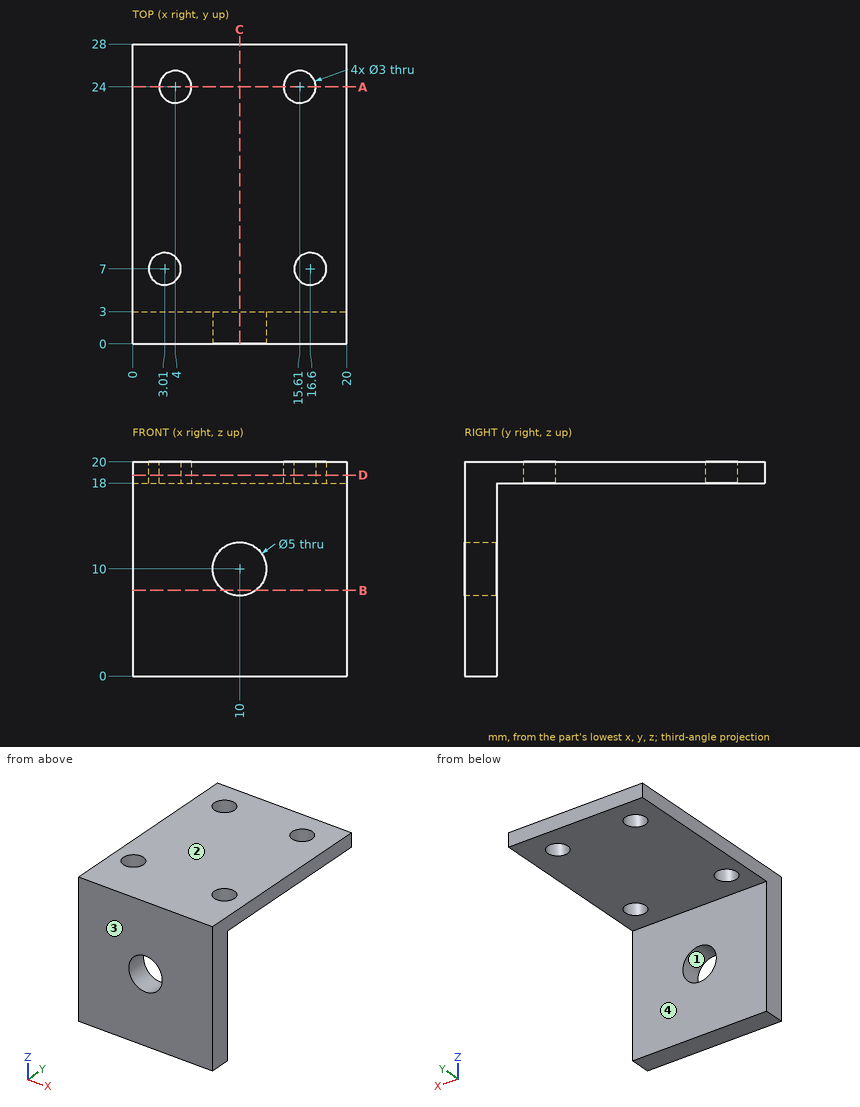
Design review of the part shown in the three views and the two pictorial views. Dimensions are in mm from the part's minimum x, y and z. A direction names the side the tool comes from. Coordinates: 2 decimals unless noted, no trailing zeros. Write each loop counter-clockwise with the first axis right and the second up, starting at its lowest first coordinate (ties: lowest second). Pieces come first, ordered by that corner, then holes. Notation, with made-up numbers: (-17, 59) -> (-7, 59) arc R16 cw to (-7, 81) -> close; hole circle Ø5 at (25.25, 76). An arc over 180 degrees is marked (long way). Answer in a Markdown table with one row per item.
1. Wall thickness on probe 1 along Y at (x, z) = (16.6, 18.65); probe 2 along X at (y, z) = (2.2, 10); probe 3 along Z at (x, y) = (3.5, 15): over which ranges is each line inside the solid? List them lowest first. Write a range as [from, to].
Answers below:
| item | result |
|---|---|
| probe 1 | y = [0, 5.5], [8.5, 22.87], [25.13, 28] |
| probe 2 | x = [0, 7.5], [12.5, 20] |
| probe 3 | z = [18, 20] |
2. For the marked faces 3 and 4, list the 3-axis set-ups (+Z, -Z, +X, -X, +Y, -Y) from which the entire face can be reached by the end or side of a thin tool; tool diameter is ignored.
Answers below:
| item | result |
|---|---|
| face 3 | +Z, -Z, +X, -X, -Y |
| face 4 | -Z, +X, -X, +Y |
3. We need section D-D, the plane z = 18.75. State the section outline as (x, y) points.
Answers below:
| item | result |
|---|---|
| outline | (0, 0) -> (20, 0) -> (20, 28) -> (0, 28) -> close; hole circle Ø3 at (3.01, 7); hole circle Ø3 at (4, 24); hole circle Ø3 at (15.61, 24); hole circle Ø3 at (16.6, 7) |
4. Clearance check with flat-ended pins moving along their axes: pin 1 Ø1.5 at (x, z) = (8, 10.5) entering from +Y; pin 2 Ø5 at (x, y) = (5, 24.5) entering from -Z. State where each tip first meets the part, or that it passes through.
Answers below:
| item | result |
|---|---|
| pin 1 | stops at y = 3 |
| pin 2 | stops at z = 18 |
5. We need section A-A, the plane y = 24. State the section outline as (x, z) points.
Answers below:
| item | result |
|---|---|
| outline | (0, 18) -> (2.5, 18) -> (2.5, 20) -> (0, 20) -> close; (5.5, 18) -> (14.11, 18) -> (14.11, 20) -> (5.5, 20) -> close; (17.11, 18) -> (20, 18) -> (20, 20) -> (17.11, 20) -> close |
6. We need section C-C, the plane x = 10. State the section outline as (y, z) points, and give its area (3 significant figures).
Answers below:
| item | result |
|---|---|
| outline | (0, 0) -> (3, 0) -> (3, 7.5) -> (0, 7.5) -> close; (0, 12.5) -> (3, 12.5) -> (3, 18) -> (28, 18) -> (28, 20) -> (0, 20) -> close |
| area | 95.0 mm^2 |
7. We need section B-B, the plane z = 8. State the section outline as (x, y) points.
Answers below:
| item | result |
|---|---|
| outline | (0, 0) -> (8.5, 0) -> (8.5, 3) -> (0, 3) -> close; (11.5, 0) -> (20, 0) -> (20, 3) -> (11.5, 3) -> close |
8. Draft analysis for pull direction X (two halves, no side actions). For the marked faces 1 and 2, state which applies: +X half, -X half, draft (parallel to the pull), parting line (faces both ways), or undercut.
Answers below:
| item | result |
|---|---|
| face 1 | undercut |
| face 2 | draft |
